Can you work these out from the drawing? Everything is in mm from the part's minimum corner. Coordinates: 2 decimals unless noted, no trailing zeros. Loops run counter-clockwise (first coordinate to the right, second up) from the corner with the lowest first, then second, coordinate; pieces in that order, holes last. Notation, with made-up numbers: (-9, -23.5) -> (-5, -23.5) arc R12 cw to (-5, -8.5) -> close; hole circle Ø11 at (-39, 78.5). An arc over 180 degrees is marked (long way). Put each result on its own line as item: value. Start each with the question number.
Item 1: Will this pin go through, and if not, where does the flat tip stop? P1, Ø5, axis at x = 25, y = 17, coming from the -Z side.
Item 2: Please list where these lines run through material, in increasing order: L1, parallel to X at y = 29, z = 42 (1 decimal); L2, parallel to X at y = 8.5, z = 32 (1 decimal); L3, parallel to Y at x = 35.5, z = 29. Write a range as from..to.
Item 3: If we section it at D-D on x = 83.5: Please give me the cut outline in (y, z), plus the area to 3 significant figures.
Item 4: We'd pull the mould along X, two halves only. Please class the marked faces 1, 2, 3 and 4: pulls with the +X half, pulls with the -X half, needs draft (parallel to the pull), parting line crosses it, or undercut.
Item 5: If we section it at A-A on y = 10.5: Please give me the cut outline in (x, z) (1 decimal), plus the area to 3 significant figures.
Item 6: If we section it at B-B on z = 19.5: Please give me the cut outline in (x, y) (1 decimal), plus the area to 3 significant figures.
Item 7: If we section it at C-C on y = 5: Please give me the cut outline in (x, z) (1 decimal), plus the area to 3 significant figures.
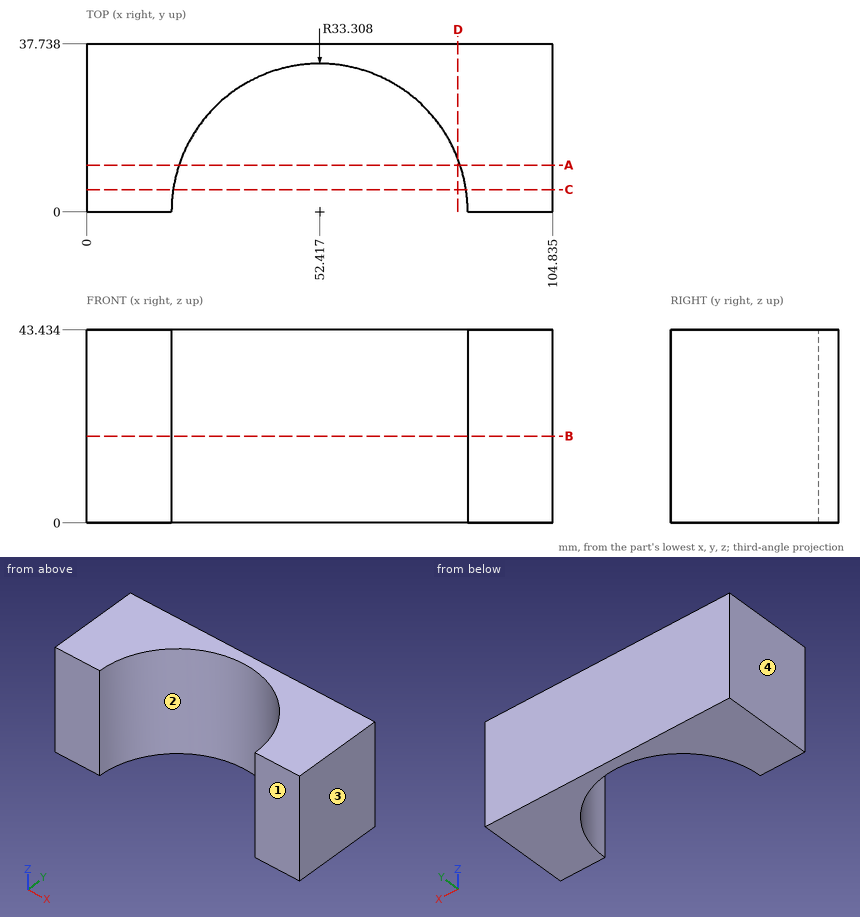
Solutions:
1. P1: z = 0
2. L1: 0..36, 68.8..104.8
2. L2: 0..20.2, 84.6..104.8
2. L3: 28.69..37.74
3. outline: (11.97, 0) -> (37.74, 0) -> (37.74, 43.43) -> (11.97, 43.43) -> close
3. area: 1,120 mm^2
4. face 1: needs draft
4. face 2: undercut
4. face 3: pulls with the +X half
4. face 4: pulls with the -X half
5. outline: (0, 0) -> (20.8, 0) -> (20.8, 43.4) -> (0, 43.4) -> close; (84, 0) -> (104.8, 0) -> (104.8, 43.4) -> (84, 43.4) -> close
5. area: 1,810 mm^2
6. outline: (0, 0) -> (19.1, 0) arc R33.3 cw to (85.7, 0) -> (104.8, 0) -> (104.8, 37.7) -> (0, 37.7) -> close
6. area: 2,210 mm^2
7. outline: (0, 0) -> (19.5, 0) -> (19.5, 43.4) -> (0, 43.4) -> close; (85.3, 0) -> (104.8, 0) -> (104.8, 43.4) -> (85.3, 43.4) -> close
7. area: 1,690 mm^2
